```python
from build123d import *

# Parameters (mm, degrees)
CYLINDER001_R     = 1.7
CYLINDER001_DEPTH = 10
CYLINDER002_R     = 1.7
CYLINDER002_DEPTH = 10
CYLINDER003_R     = 1.7
CYLINDER003_DEPTH = 10
CYLINDER_R        = 1.7
CYLINDER_DEPTH    = 10
CYLINDER010_R     = 3.2
CYLINDER010_DEPTH = 10
CYLINDER009_R     = 3.2
CYLINDER009_DEPTH = 10
CYLINDER008_R     = 3.2
CYLINDER008_DEPTH = 10
CYLINDER011_R     = 3.2
CYLINDER011_DEPTH = 10
CYLINDER005_R     = 6.2
CYLINDER005_DEPTH = 5
CYLINDER006_R     = 6.2
CYLINDER006_DEPTH = 5
CYLINDER007_R     = 6.2
CYLINDER007_DEPTH = 5
BOX_W             = 24
BOX_H             = 24
BOX_DEPTH         = 5
CYLINDER004_R     = 6.2
CYLINDER004_DEPTH = 5
CHAMFER_SIZE      = 0.4
CHAMFER001_SIZE   = 0.4


with BuildPart() as cylinder001:
    # Cylinder001 → Cylinder001 (new body)
    with BuildSketch(Plane(origin=(-7.75, 7.75, 0), x_dir=(1, 0, 0), z_dir=(0, 0, 1))):
        Circle(CYLINDER001_R)
    extrude(amount=CYLINDER001_DEPTH)


with BuildPart() as cylinder002:
    # Cylinder002 → Cylinder002 (new body)
    with BuildSketch(Plane(origin=(7.75, -7.75, 0), x_dir=(1, 0, 0), z_dir=(0, 0, 1))):
        Circle(CYLINDER002_R)
    extrude(amount=CYLINDER002_DEPTH)


with BuildPart() as cylinder003:
    # Cylinder003 → Cylinder003 (new body)
    with BuildSketch(Plane(origin=(-7.75, -7.75, 0), x_dir=(1, 0, 0), z_dir=(0, 0, 1))):
        Circle(CYLINDER003_R)
    extrude(amount=CYLINDER003_DEPTH)


with BuildPart() as fusion002:
    # Cylinder → Cylinder (new body)
    with BuildSketch(Plane(origin=(7.75, 7.75, 0), x_dir=(1, 0, 0), z_dir=(0, 0, 1))):
        Circle(CYLINDER_R)
    extrude(amount=CYLINDER_DEPTH)

    # Fusion002: union Cylinder001, Cylinder002, Cylinder003
    add(cylinder001.part)
    add(cylinder002.part)
    add(cylinder003.part)


with BuildPart() as cylinder010:
    # Cylinder010 → Cylinder010 (new body)
    with BuildSketch(Plane(origin=(-7.75, 7.75, 0), x_dir=(1, 0, 0), z_dir=(0, 0, 1))):
        Circle(CYLINDER010_R)
    extrude(amount=CYLINDER010_DEPTH)


with BuildPart() as cylinder009:
    # Cylinder009 → Cylinder009 (new body)
    with BuildSketch(Plane(origin=(7.75, 7.75, 0), x_dir=(1, 0, 0), z_dir=(0, 0, 1))):
        Circle(CYLINDER009_R)
    extrude(amount=CYLINDER009_DEPTH)


with BuildPart() as cylinder008:
    # Cylinder008 → Cylinder008 (new body)
    with BuildSketch(Plane(origin=(-7.75, -7.75, 0), x_dir=(1, 0, 0), z_dir=(0, 0, 1))):
        Circle(CYLINDER008_R)
    extrude(amount=CYLINDER008_DEPTH)


with BuildPart() as fusion:
    # Cylinder011 → Cylinder011 (new body)
    with BuildSketch(Plane(origin=(7.75, -7.75, 0), x_dir=(1, 0, 0), z_dir=(0, 0, 1))):
        Circle(CYLINDER011_R)
    extrude(amount=CYLINDER011_DEPTH)

    # Fusion: union Cylinder010, Cylinder009, Cylinder008
    add(cylinder010.part)
    add(cylinder009.part)
    add(cylinder008.part)


with BuildPart() as fusion_1:
    # Fusion placement: moved
    add(fusion.part.moved(Location((0, 0, 3))))


with BuildPart() as cylinder005:
    # Cylinder005 → Cylinder005 (new body)
    with BuildSketch(Plane(origin=(7.75, -7.75, 0), x_dir=(1, 0, 0), z_dir=(0, 0, 1))):
        Circle(CYLINDER005_R)
    extrude(amount=CYLINDER005_DEPTH)


with BuildPart() as cylinder006:
    # Cylinder006 → Cylinder006 (new body)
    with BuildSketch(Plane(origin=(-7.75, 7.75, 0), x_dir=(1, 0, 0), z_dir=(0, 0, 1))):
        Circle(CYLINDER006_R)
    extrude(amount=CYLINDER006_DEPTH)


with BuildPart() as cylinder007:
    # Cylinder007 → Cylinder007 (new body)
    with BuildSketch(Plane(origin=(7.75, 7.75, 0), x_dir=(1, 0, 0), z_dir=(0, 0, 1))):
        Circle(CYLINDER007_R)
    extrude(amount=CYLINDER007_DEPTH)


with BuildPart() as cube:
    # Box → Box (new body)
    with BuildSketch(Plane(origin=(-12, -12, 0), x_dir=(1, 0, 0), z_dir=(0, 0, 1))):
        with Locations((12, 12)):
            Rectangle(BOX_W, BOX_H)
    extrude(amount=BOX_DEPTH)


with BuildPart() as chamfer001001:
    # Cylinder004 → Cylinder004 (new body)
    with BuildSketch(Plane(origin=(-7.75, -7.75, 0), x_dir=(1, 0, 0), z_dir=(0, 0, 1))):
        Circle(CYLINDER004_R)
    extrude(amount=CYLINDER004_DEPTH)

    # Fusion001: union Cylinder005, Cylinder006, Cylinder007, Cube
    add(cylinder005.part)
    add(cylinder006.part)
    add(cylinder007.part)
    add(cube.part)

    # Cut: cut Fusion
    add(fusion_1.part, mode=Mode.SUBTRACT)

    # Cut001: cut Fusion002
    add(fusion002.part, mode=Mode.SUBTRACT)

    # Chamfer
    chamfer_edges = [chamfer001001.edges().sort_by_distance(p)[0] for p in [
        (0, -12, 5),
        (-12.134062, -12.134062, 5),
        (-12, 0, 5),
        (-12.134062, 12.134062, 5),
        (0, 12, 5),
        (12, 0, 5),
        (-10.95, -7.75, 5),
        (4.55, -7.75, 5),
        (-10.95, 7.75, 5),
        (4.55, 7.75, 5),
        (10.036078, -13.513146, 5),
        (13.441661, -5.291342, 5),
        (13.441661, 5.291342, 5),
        (10.036078, 13.513146, 5),
    ]]
    chamfer(chamfer_edges, length=CHAMFER_SIZE)

    # Chamfer001
    chamfer001_edges = [chamfer001001.edges().sort_by_distance(p)[0] for p in [
        (0, -12, 0),
        (10.036078, -13.513146, 0),
        (13.441661, -5.291342, 0),
        (-12, 0, 0),
        (-12.134062, 12.134062, 0),
        (0, 12, 0),
        (10.036078, 13.513146, 0),
        (13.441661, 5.291342, 0),
        (12, 0, 0),
        (-12.134062, -12.134062, 0),
        (-9.45, -7.75, 0),
        (6.05, -7.75, 0),
        (-9.45, 7.75, 0),
        (6.05, 7.75, 0),
    ]]
    chamfer(chamfer001_edges, length=CHAMFER001_SIZE)


solid = chamfer001001.part
```
Design review of the part built by this model. Coordinates are the model's own, in mm. A direction names the side the tool comes from. Give positions to 0.01 mm unless a question says otherwise; leave off trailing zeros. Write each loop counter-clockwise with the first axis right and the second up, starting at its lowest first coordinate (ties: lowest second). Pieces come first, ordered by that corner, then holes. Notation, with made-up numbers: (75.5, -27.75) - (82.5, -27.75) arc R25 cw to (82.5, 6.25) - close; hole circle Ø6 at (12, -34). An arc over 180 degrees is marked (long way). Return JSON: item names as keys, results as strings. Group by question number.
(1) Insertion check: pin 1 (8.5 mm diameter, centred on x = -7.75, y = 7.75, fed in from -Z); pin 2 (1.5 mm diameter, centred on y = 1.5, z = 1, fed in from +X); pin 3 (4 mm diameter, centred on x = -7.75, y = -7.75, fed in from +Z); pin 4 (4 mm diameter, centred on x = 7.75, y = 7.75, fed in from -Z). Each pin has a flat end and moves straight along its axis. Give the tip position at first contact, or say it passes through.
(2) We need section D-D, the plane x = 1. Give the boundary of the cut face in (y, z), then the cut area to 3 significant figures.
(3) To check wall thickness, follow probe 1 along Y at (x, z) = (-7.75, 1.35); probe 2 along Y at (x, z) = (7.75, 3.95). State the ranges of each line that lie inside material, in increasing order.
(4) Machinability: for faces 1 (the flat face through (-12, 0, 2)), 2 (the cylindrical face through (9.227, 4.911, 3.789)), 3 (the flat face through (0, 12, 2)), which of the approach directions +Z, -Z, +X, -X, +Y, -Y give a long, thin tool a straight path to every point of the face, cutting with its end or side? Answer none if there is none.
(5) We need section A-A, the plane y = -7.75. Give the number of separate pieces and of enclosed holes in the cut face, then the cut area to 3 significant figures.
(6) Mouldability with a two-part tool opening along Y and no side actions: class faces 4 (the conical face through (11.835, 12.026, 0.114)), 5 (the flat face through (0, 0, 0)), 6 (the flat face through (0, -12, 2)), 7 (the cylindrical face through (6.05, 7.82, 1.68)) as +Y half, -Y half, draft (parallel to the pull), parting line (faces both ways), or undercut.
Reported:
{
 "1": {"pin 1": "stops at z = 0", "pin 2": "stops at x = 12", "pin 3": "stops at z = 3", "pin 4": "stops at z = 0.1"},
 "2": {"outline": "(-12, 0.4) - (-11.6, 0) - (11.6, 0) - (12, 0.4) - (12, 4.6) - (11.6, 5) - (-11.6, 5) - (-12, 4.6) - close", "area": "120 mm2"},
 "3": {"probe 1": "y = -13.95 to -9.45, -6.05 to 6.05, 9.45 to 13.95", "probe 2": "y = -13.95 to -10.95, -4.55 to 4.55, 10.95 to 13.95"},
 "4": {"face 1": "+Z, -Z, -X", "face 2": "+Z", "face 3": "+Z, -Z, +Y"},
 "5": {"separate pieces": "3", "enclosed holes": "0", "area": "92.5 mm2"},
 "6": {"face 4": "undercut", "face 5": "draft", "face 6": "-Y half", "face 7": "undercut"}
}
